from build123d import *

# Parameters (mm, degrees)
SKETCH1_R           = 2.794
BOSS_EXTRUDE1_DEPTH = 4.6355
SKETCH2_W           = 10.4775
SKETCH2_H           = 9.271
BOSS_EXTRUDE2_DEPTH = 2.54
SKETCH3_W           = 7.8105
SKETCH3_H           = 10.4775
BOSS_EXTRUDE3_DEPTH = 7.366
SKETCH4_W           = 3.302
SKETCH4_H           = 6.604
CUT_EXTRUDE1_DEPTH  = 10.4775
SKETCH5_R           = 1.651
CUT_EXTRUDE2_DEPTH  = 15.8115
FILLET1_R           = 0.762


with BuildPart() as part:
    # Sketch1 → Boss-Extrude1 (new body, symmetric)
    with BuildSketch(Plane(origin=(0, 0, 0), x_dir=(1, 0, 0), z_dir=(0, 1, 0))):
        Polygon((-11.1125, 3.81), (-4.191, 3.81), (-4.191, 9.144), (14.2875, 9.144), (14.2875, -6.6675), (-11.1125, -6.6675), align=None)
        Circle(SKETCH1_R, mode=Mode.SUBTRACT)
    extrude(amount=BOSS_EXTRUDE1_DEPTH, both=True)

    # Sketch2 → Boss-Extrude2 (add)
    with BuildSketch(Plane.ZY.offset(11.1125)):
        with Locations((1.42875, 0)):
            Rectangle(SKETCH2_W, SKETCH2_H)
    extrude(amount=BOSS_EXTRUDE2_DEPTH)

    # Sketch3 → Boss-Extrude3 (add, symmetric)
    with BuildSketch(Plane(origin=(0, 0, 0), x_dir=(1, 0, 0), z_dir=(0, 1, 0))):
        with Locations((-9.74725, -1.42875)):
            Rectangle(SKETCH3_W, SKETCH3_H)
    extrude(amount=BOSS_EXTRUDE3_DEPTH, both=True)

    # Sketch4 → Cut-Extrude1 (cut)
    with BuildSketch(Plane(origin=(0, 0, -3.81), x_dir=(-1, 0, 0), z_dir=(0, 0, -1))):
        with Locations((8.636, 0)):
            Rectangle(SKETCH4_W, SKETCH4_H)
    extrude(amount=-CUT_EXTRUDE1_DEPTH, mode=Mode.SUBTRACT)

    # Sketch5 → Cut-Extrude2 (cut)
    with BuildSketch(Plane.XY.offset(6.6675)):
        with Locations((9.2075, 0)):
            Circle(SKETCH5_R)
    extrude(amount=-CUT_EXTRUDE2_DEPTH, mode=Mode.SUBTRACT)

    # Fillet1
    fillet1_edges = [part.edges().sort_by_distance(p)[0] for p in [
        (14.2875, 4.6355, -1.23825),
        (-4.191, 0, -3.81),
        (-4.191, 0, -9.144),
        (14.2875, 0, -9.144),
        (14.2875, 0, 6.6675),
        (5.04825, 4.6355, -9.144),
        (-4.191, 4.6355, -6.477),
        (-5.0165, 4.6355, -3.81),
        (-13.6525, 0, -3.81),
        (-13.6525, 0, 6.6675),
        (4.22275, -4.6355, 6.6675),
        (4.22275, 4.6355, 6.6675),
        (-5.842, 6.00075, 6.6675),
        (-5.842, 6.00075, -3.81),
        (-5.842, -6.00075, 6.6675),
        (-5.842, -7.366, 1.42875),
        (-5.842, -6.00075, -3.81),
        (-9.74725, -7.366, -3.81),
        (-13.6525, -7.366, 1.42875),
        (-9.74725, -7.366, 6.6675),
        (-5.842, 7.366, 1.42875),
        (-9.74725, 7.366, -3.81),
        (-13.6525, 7.366, 1.42875),
        (-9.74725, 7.366, 6.6675),
        (-5.0165, -4.6355, -3.81),
        (-4.191, -4.6355, -6.477),
        (5.04825, -4.6355, -9.144),
        (14.2875, -4.6355, -1.23825),
    ]]
    fillet(fillet1_edges, radius=FILLET1_R)


solid = part.part
Could you check a few things on this model? Use its own coordinates, in mm. A direction names the side the tool comes from. Give positions to 0.01 mm unless a question says otherwise; leave off trailing zeros. Loops run counter-clockwise (first coordinate to the right, second up) from the corner with the lowest first, then second, coordinate; pieces in that order, holes last. Notation, with made-up numbers: (29, 28) -> (62, 28) arc R19 ccw to (62, 48) -> close; hole circle Ø5 at (-23.5, 49.25). An arc over 180 degrees is marked (long way). Return JSON: item names as keys, results as strings.
Item 1: Which directions (+Z, -Z, +X, -X, +Y, -Y) give clear straight access to the entire face, cutting with the end or side of a thin tool? Please do faces 5 (the flat face through (-4.191, 0, -6)), 6 (the flat face through (-10.287, 0, 1)), 7 (the flat face through (4, -4.636, -1)), 8 (the flat face through (-5.842, 6, 1)), 9 (the flat face through (-10, -7.366, 1)).
Geometry results:
{"face 5": "-Z, -X, +Y, -Y", "face 6": "+Z, -Z", "face 7": "+Z, -Z, +X, -Y", "face 8": "+Z, -Z, +X, +Y", "face 9": "+Z, -Z, +X, -X, -Y"}
Item 2: We'd pull the mould along X, two halves only. Please class faces 1 (the flat face through (-9, 3.302, 1)), 2 (the flat face through (-10, 7.366, 1)), 3 (the flat face through (-5.842, -6, 1)), 4 (the flat face through (-9, -3.302, 1)): +X half, -X half, draft (parallel to the pull), parting line (faces both ways), or undercut.
Geometry results:
{"face 1": "undercut", "face 2": "draft", "face 3": "+X half", "face 4": "undercut"}
Item 3: If we section it at C-C on y = -2.75: List the corners of the cut face in (x, z) for me (1 decimal).
Geometry results:
{"outline": "(-13.7, -3) arc R0.8 ccw to (-12.9, -3.8) -> (-10.3, -3.8) -> (-10.3, 6.7) -> (-12.9, 6.7) arc R0.8 ccw to (-13.7, 5.9) -> close; (-7, -3.8) -> (-5, -3.8) arc R0.8 cw to (-4.2, -4.6) -> (-4.2, -8.4) arc R0.8 ccw to (-3.4, -9.1) -> (13.5, -9.1) arc R0.8 ccw to (14.3, -8.4) -> (14.3, 5.9) arc R0.8 ccw to (13.5, 6.7) -> (-7, 6.7) -> close; hole circle Ø5.6 at (0, 0)"}
Item 4: I need wall thicknesses on L1, parallel to X at y = -1.75, z = 0 (1 decimal); L2, parallel to Y at x = -10.25, z = 1.5; L3, parallel to X at y = 0.5, z = 1.75 (1 decimal). Which ranges of each line are inside material? Lowest first, please. Write a range as from..to.
Geometry results:
{"L1": "x = -13.7..-10.3, -7..-2.8, 2.8..14.3", "L2": "y = -7.37..-3.3, 3.3..7.37", "L3": "x = -13.7..-10.3, -7..-2.2, 2.2..7.6, 10.8..14.3"}
Item 5: If we section it at D-D on z = 0: List the corners of the cut face in (x, y) for me (1 decimal).
Geometry results:
{"outline": "(-13.7, -6.6) arc R0.8 ccw to (-12.9, -7.4) -> (-6.6, -7.4) arc R0.8 ccw to (-5.8, -6.6) -> (-5.8, -4.6) -> (-2.8, -4.6) -> (-2.8, 4.6) -> (-5.8, 4.6) -> (-5.8, 6.6) arc R0.8 ccw to (-6.6, 7.4) -> (-12.9, 7.4) arc R0.8 ccw to (-13.7, 6.6) -> close; (2.8, -4.6) -> (13.5, -4.6) arc R0.8 ccw to (14.3, -3.9) -> (14.3, 3.9) arc R0.8 ccw to (13.5, 4.6) -> (2.8, 4.6) -> close; hole (-10.3, -3.3) -> (-7, -3.3) -> (-7, 3.3) -> (-10.3, 3.3) -> close; hole circle Ø3.3 at (9.2, 0)"}
Item 6: If we section it at B-B on x = -10: List the corners of the cut face in (y, z) for me.
Geometry results:
{"outline": "(-7.37, -3.05) arc R0.76 ccw to (-6.6, -3.81) -> (-3.3, -3.81) -> (-3.3, 6.67) -> (-6.6, 6.67) arc R0.76 ccw to (-7.37, 5.91) -> close; (3.3, -3.81) -> (6.6, -3.81) arc R0.76 ccw to (7.37, -3.05) -> (7.37, 5.91) arc R0.76 ccw to (6.6, 6.67) -> (3.3, 6.67) -> close"}
Item 7: If we section it at A-A on y = 0: List the corners of the cut face in (x, z) for me (1 decimal), plus the area to 3 significant figures.
Geometry results:
{"outline": "(-13.7, -3) arc R0.8 ccw to (-12.9, -3.8) -> (-10.3, -3.8) -> (-10.3, 6.7) -> (-12.9, 6.7) arc R0.8 ccw to (-13.7, 5.9) -> close; (-7, -3.8) -> (-5, -3.8) arc R0.8 cw to (-4.2, -4.6) -> (-4.2, -8.4) arc R0.8 ccw to (-3.4, -9.1) -> (7.6, -9.1) -> (7.6, 6.7) -> (-7, 6.7) -> close; (10.9, -9.1) -> (13.5, -9.1) arc R0.8 ccw to (14.3, -8.4) -> (14.3, 5.9) arc R0.8 ccw to (13.5, 6.7) -> (10.9, 6.7) -> close; hole circle Ø5.6 at (0, 0)", "area": "279 mm²"}
Item 8: I'm going to push flat-ended pins straight in: pin 1 (2.5 mm diameter, centred on x = -10.5, y = -0.5, fed in from -Z); pin 2 (7.5 mm diameter, centred on x = 0, z = 0, fed in from -Y); pin 3 (4 mm diameter, centred on y = 1.5, z = -6, fed in from -X). Where does each tip first touch, or does it pass through?
Geometry results:
{"pin 1": "stops at z = -3.81", "pin 2": "stops at y = -4.64", "pin 3": "stops at x = -4.45"}
